```python
from build123d import *

# Parameters (mm, degrees)
F2_W     = 4.05
F2_H     = 8.1
F3_DEPTH = 6
F4_R     = 0.75
F5_R     = 2
F6_R     = 0.5


with BuildPart() as f1:
    # F0 (on Front) → F1 (revolve)
    with BuildSketch(Plane.XZ):
        Polygon((4.05, 0), (4.05, 6), (5.5, 7), (10.5, 7), (9.5900744143, 9.5), (7.5900744143, 9.5), (4.991998203, 8), (0, 8), (0, 0), align=None)
    revolve(axis=Axis((0, 0, 4), (0, 0, -1)))

    # F2 (on face) → F3 (cut)
    with BuildSketch(Plane(origin=(0, 0, 0), x_dir=(1, 0, 0), z_dir=(0, 0, -1))):
        with Locations((2.025, 0)):
            Rectangle(F2_W, F2_H)
    extrude(amount=-F3_DEPTH, mode=Mode.SUBTRACT)

    # F4
    f4_edges = [f1.edges().sort_by_distance(p)[0] for p in [
        (0, 0, 0),
        (0, 0, 6),
        (-4.05, 0, 0),
    ]]
    fillet(f4_edges, radius=F4_R)

    # F5
    f5_edges = [f1.edges().sort_by_distance(p)[0] for p in [
        (-9.590074, 0, 9.5),
        (-7.590074, 0, 9.5),
        (-4.991998, 0, 8),
    ]]
    fillet(f5_edges, radius=F5_R)

    # F6
    f6_edges = [f1.edges().sort_by_distance(p)[0] for p in [
        (-10.5, 0, 7),
    ]]
    fillet(f6_edges, radius=F6_R)


solid = f1.part
```
Design review of the part built by this model. Coordinates are the model's own, in mm. A direction names the side the tool comes from. Give positions to 0.01 mm unless a question says otherwise; leave off trailing zeros. Loops run counter-clockwise (first coordinate to the right, second up) from the corner with the lowest first, then second, coordinate; pieces in that order, holes last. Notation, with made-up numbers: (5.25, -9.5) -> (61.25, -9.5) arc R32 ccw to (61.25, 25.5) -> close; hole circle Ø8 at (-21, 82.5). An arc over 180 degrees is marked (long way). Write each question's results on one line, items separated by ' | '.
Q1. Wall thickness on L1, parallel to X at y = 2, z = 8.75; L2, parallel to Z at x = -0.25, y = -5; L3, parallel to X at y = 8.25, z = 8.25: over which ranges is each line inside the solid? List them lowest first.
Reply:
L1: x = -9.54 to -5.96, 5.96 to 9.54 | L2: z = 6.66 to 8.08 | L3: x = -5.73 to 5.73
Q2. For pin 1 Ø1 at (x, y) = (2.5, 2) entering from -Z; pin 2 Ø2 at (x, y) = (-7, -6.5) entering from +Z; pin 3 Ø2 at (y, z) = (-1, 2.5) entering from +X, all flat-tipped, find the tip position at first contact; note any pin that passes through.
Reply:
pin 1: stops at z = 6 | pin 2: stops at z = 9.47 | pin 3: stops at x = 0
Q3. Take a section at A-A, the plane y = 0. Write out the cut boundary in (x, z), plus the area to 3 significant figures.
Reply:
outline: (-10.26, 7.67) arc R0.5 ccw to (-9.79, 7) -> (-5.5, 7) -> (-4.05, 6) -> (-4.05, 0.75) arc R0.75 ccw to (-3.3, 0) -> (-0.75, 0) arc R0.75 ccw to (0, 0.75) -> (0, 5.25) arc R0.75 cw to (0.75, 6) -> (4.05, 6) -> (5.5, 7) -> (9.79, 7) arc R0.5 ccw to (10.26, 7.67) -> (10.07, 8.18) arc R2 ccw to (8.19, 9.5) -> (8.13, 9.5) arc R2 ccw to (7.13, 9.23) -> (5.46, 8.27) arc R2 cw to (4.46, 8) -> (-4.46, 8) arc R2 cw to (-5.46, 8.27) -> (-7.13, 9.23) arc R2 ccw to (-8.13, 9.5) -> (-8.19, 9.5) arc R2 ccw to (-10.07, 8.18) -> close | area: 64.1 mm²
Q4. Machinability: for faces 1 (the face through (-2, 0, 0)), 2 (the face through (2, 0, 6)), which of the approach directions +Z, -Z, +X, -X, +Y, -Y give a long, thin tool a straight path to every point of the face, cutting with its end or side? Answer none if there is none.
Reply:
face 1: -Z, +X, -X, +Y, -Y | face 2: -Z, +X, +Y, -Y
Q5. Take a section at B-B, the plane z = 2.5. Write out the cut boundary in (x, y).
Reply:
outline: (0, -4.05) -> (0, 4.05) arc R4.05 ccw to start
Q6. The part is to be moulded in two halves that separate along X. For faces 3 (the face through (0, 0, 3)), 4 (the face through (-4, 4, 7)), 5 (the face through (0, 0, 8)), say which applies: +X half, -X half, draft (parallel to the pull), parting line (faces both ways), or undercut.
Reply:
face 3: +X half | face 4: draft | face 5: undercut
